Autodesk Fusion 360 part; units mm, degrees
sketch "Sketch1" plane through (0, 0, 0) normal (0, 0, 1) x (1, 0, 0)
  circle A0 centre (0, 0) radius 2.45
  dimension "d1" = 4.9
extrude "Extrude1" add sketch "Sketch1" along normal blind 70
sketch "Sketch2" plane through (0, 0, 0) normal (0, 0, 1) x (1, 0, 0)
  line L0 (0, 0) -> (2.45, 0)
  line L1 (2.45, 0) -> (-2.45, 0)
  line L2 (-2.45, 0) -> (-2.45, 2.45)
  line L3 (-2.45, 2.45) -> (2.45, 2.45)
  line L4 (2.45, 2.45) -> (2.45, 0)
  dimension "d4" = 2.45
  dimension "d5" = 4.9
  dimension "d6" = 2.45
extrude "Extrude2" add sketch "Sketch2" along normal blind 11
sketch "Sketch3" plane through (0, 2.45, 0) normal (0, 1, 0) x (-1, 0, 0)
  line L0 (0, 11) -> (-2.45, 11)
  line L1 (-2.45, 11) -> (-2.45, 0)
  line L2 (-2.45, 0) -> (2.45, 0)
  line L3 (2.45, 0) -> (2.45, 11)
  line L4 (2.45, 11) -> (0, 11)
  line L5 (2.45, 0) -> (-2.45, 0)
  line L6 (-2.45, 0) -> (-2.45, 1.6)
  line L7 (-2.45, 1.6) -> (2.45, 1.6)
  line L8 (2.45, 1.6) -> (2.45, 0)
  dimension "d9" = 1.6
extrude "Extrude3" add sketch "Sketch3" along normal blind 1 contours L1 L2 L3 L5 L6 L7 L8
sketch "Sketch4" plane through (0, 0, 0) normal (1, 0, 0) x (0, 0, -1)
  line L0 (0, 0) -> (0, -2.45)
  line L1 (0, -2.45) -> (-6.9, -2.45)
  line L2 (-6.9, -2.45) -> (-4.9, -2.45)
  line L3 (-5.9, -2.45) -> (-5.9, -1.825)
  line L4 (-5.9, -1.825) -> (-5.9, -1.325)
  line L5 (-5.9, -1.325) -> (-5.9, -1.2)
  line L6 (0, 0) -> (-0.3154, 0)
  line L7 (-0.3154, 0) -> (-5.9, 0)
  line L8 (-5.9, 0) -> (-2.9, 0)
  line L9 (-5.9, 0) -> (-8.9, 0)
  line L10 (-8.9, 0) -> (-2.9, 0) construction
  line L11 (-1.7, 0) -> (-10.1, 0)
  line L12 (-2.9, 1.575) -> (-8.9, 1.575)
  arc A0 (-8.9, 1.575) -> (-8.9, -1.575) centre (-8.9, 0) ccw
  line L13 (-8.9, -1.575) -> (-2.9, -1.575)
  arc A1 (-2.9, -1.575) -> (-2.9, 1.575) centre (-2.9, 0) ccw
  line L14 (-2.9, 0) -> (-8.9, 0) construction
  line L15 (-10.1, 0) -> (-10.475, 0)
  ellipse E0 centre (-5.9, -2.45) end of major axis (-6.9, -2.45) minor radius 0.5
  line L16 (-4.9, -2.45) -> (-6.9, -2.45) construction
  line L17 (-5.9, -1.95) -> (-5.9, -2.95) construction
  dimension "d12" = 2.45
  dimension "d13" = 6.9
  dimension "d14" = 2
  dimension "d16" = 0.5
  dimension "d17" = 3
  dimension "d18" = 3
  dimension "d29" = 1
extrude "Extrude4" [suppressed]
extrude "Extrude5" [suppressed]
sketch "Sketch5" plane through (0, 0, 70) normal (0, 0, 1) x (1, 0, 0)
  circle A0 centre (0, 0) radius 2.45
  circle A1 centre (0, 0) radius 1.5
extrude "Extrude6" [suppressed]
fillet "Fillet1" [suppressed]
chamfer "Chamfer1" [suppressed]
moveface "MoveFace1" [suppressed]
fillet "Fillet2" [suppressed]
fillet "Fillet3" [suppressed]
move_face "OffsetFaces1" [suppressed]
moveface "MoveFace2" [suppressed]
sketch "Sketch6" plane through (0, 0, 0) normal (0, 0, 1) x (1, 0, 0)
  circle A0 centre (0, 0) radius 2.45
  line L0 (0, 0) -> (0, -2.45)
  line L1 (0, -2.45) -> (0, -2.95)
  line L2 (0, -2.95) -> (-0.5, -2.95)
  line L3 (-0.5, -2.95) -> (-0.5, -2.3984)
  line L4 (-0.5, -2.3984) -> (0, -2.3984)
  line L5 (0, -2.3984) -> (0, -2.95)
  line L6 (-0.5, -2.95) -> (-0.2, -2.95)
  line L7 (-0.2, -2.95) -> (-1.5058, -1.9327)
  dimension "d30" = 4.9
  dimension "d31" = 0.5
  dimension "d32" = 0.5
  dimension "d33" = 0.3
move_body "Move2" [suppressed]
equation "d4 = ( 4.9 / 2 ) * 1 mm"
equation "d6 = ( 4.9 / 2 ) * 1 mm"
equation "d12 = ( 4.9 / 2 ) * 1 mm"
equation "d26 = ( 3 / 2 ) * 1 mm"
equation "d28 = ( ( 4.9 - 3 ) / 2 ) * 1 mm"
Design review of the part built by this model. Coordinates are the model's own, in mm. A direction names the side the tool comes from. Round coordinates to 2 decimals unless told otherwise and drop trailing zeros. Order: outer loops, then holes, each group sorted by start corner. A loop starts at its lowest first (then second) coordinate and runs counter-clockwise, first axis right, second up. Notation, with made-up numbers: M 47.5,-16 L 87.5,-16 A26 cw 87.5,9 Z; hole C -29,10.5 d9. An arc over 180 degrees is marked long. Put each result on its own line as item: value.
Q1. Consider section B-B (z = 4.5). State the section outline as (x, y) points, and give its area (3 significant figures).
Reported:
outline: M -2.45,0 A2.45 ccw 2.45,0 L 2.45,2.45 L -2.45,2.45 Z
area: 21.4 mm²
Q2. Consider section C-C (y = 0.8). State the section outline as (x, z) points, and give its area (3 significant figures).
Reported:
outline: M -2.45,0 L 2.45,0 L 2.45,11 L 2.32,11 L 2.32,70 L -2.32,70 L -2.32,11 L -2.45,11 Z
area: 327 mm²
Q3. Consider section A-A (x = 1.55). State the section outline as (y, z) points.
Reported:
outline: M -1.9,0 L 3.45,0 L 3.45,1.6 L 2.45,1.6 L 2.45,11 L 1.9,11 L 1.9,70 L -1.9,70 Z
Q4. Consider section D-D (z = 34.5). State the section outline as (x, y) points.
Reported:
outline: C 0,0 d4.9
Q5. Machinability: for faces 1 (the face through (-0.32, -2.43, 34.51)), 2 (the face through (2, 2, 11)), 3 (the face through (-2, 2, 11)), which of the approach directions +Z, -Z, +X, -X, +Y, -Y give a long, thin tool a straight path to every point of the face, cutting with its end or side? Answer none if there is none.
Reported:
face 1: +Z
face 2: +Z, +X, +Y
face 3: +Z, -X, +Y
Q6. Insertion check: pin 1 Ø1 at (x, z) = (1.5, 17) entering from +Y; pin 2 Ø2 at (y, z) = (-2, 53.5) entering from +X. Each pin has a flat end and moves straight along its axis. Give the tip position at first contact, or say it passes through.
Reported:
pin 1: y = 2.24
pin 2: x = 2.24
Q7. To check wall thickness, follow line 1 (Z direction, x = 0.4, y = 2.5); line 2 (Y direction, x = -0.15, z = 55.5). State the ranges of each line that lie inside material, in increasing order.
Reported:
line 1: 0 to 1.6
line 2: -2.45 to 2.45
